For this review, take the finished solid that the model builds, in its own axes (mm). A direction names the side the tool comes from. Give positions to 0.01 mm unless a question says otherwise; leave off trailing zeros. Loops run counter-clockwise (first coordinate to the right, second up) from the corner with the lowest first, then second, coordinate; pieces in that order, holes last. Notation, with made-up numbers: (54.25, 20.25) -> (64.25, 20.25) arc R28 ccw to (64.25, 46.25) -> close; hole circle Ø8 at (43, 71.25). An arc over 180 degrees is marked (long way). One line per question, with ' | ' between items. Start each with the question number.
(1) Consider section D-D (z = 57). Write out the cut boundary in (x, y), and give its area (3 significant figures).
(2) Consider section B-B (x = -69). Write out the cut boundary in (y, z), and give its area (3 significant figures).
(3) Tool access review of faces 1 (the flat face through (-94.5, 38, 48)), 2 (the flat face through (-44, 30, 42)): name each direction out of +Z, -Z, +X, -X, +Y, -Y from which nothing blocks a thin tool from reaching the whole face with its end or side.
(4) Insertion check: P1, Ø12, axis at x = -35, y = 38.5, coming from the +Z side. The pin has a flat end and moves straight along its axis. Give the tip position at first contact, or say it passes through.
(5) Wall thickness on probe 1 along X at (y, z) = (80.5, 51.5); probe 2 along X at (y, z) = (29, 38); probe 3 along Y at (x, z) = (-86, 50.5): over which ranges is each line inside the solid? List them lowest first.
(6) Consider section C-C (y = 68). Write out the cut boundary in (x, z), and give its area (3 significant figures).
(7) Draft analysis for pull direction Y (two halves, no side actions). For faces 3 (the flat face through (0.5, 38, 48)), 4 (the flat face through (-93.5, 48, 51)), 5 (the flat face through (-48, -6, 48)), 6 (the flat face through (-48, 84, 48)), state which applies: +Y half, -Y half, draft (parallel to the pull), parting line (faces both ways), or undercut.
(8) Consider section A-A (z = 43.5). Write out the cut boundary in (x, y), and give its area (3 significant figures).
from build123d import *

# Parameters (mm, degrees)
SKETCH017_W    = 95
SKETCH017_H    = 90
PAD010_DEPTH   = 25
THICKNESS001_T = -1
SKETCH021_W    = 50
SKETCH021_H    = 70
PAD013_DEPTH   = 10


with BuildPart() as part:
    # Sketch017 → Pad010 (new body)
    with BuildSketch(Plane.XY):
        Rectangle(SKETCH017_W, SKETCH017_H)
    extrude(amount=PAD010_DEPTH)

    # Thickness001
    thickness001_openings = [part.faces().sort_by_distance(p)[0] for p in [
        (0, 0, 25),
    ]]
    offset(amount=THICKNESS001_T, openings=thickness001_openings)

    # Sketch021 (on DatumPlane) → Pad013 (join)
    with BuildSketch(Plane.XY.offset(1)):
        with Locations((-22, -9)):
            Rectangle(SKETCH021_W, SKETCH021_H)
    extrude(amount=PAD013_DEPTH)


with BuildPart() as part_1:
    # Body005 placement: moved
    add(part.part.moved(Location((-47, 39, 36))))


solid = part_1.part
A:
1) outline: (-94.5, -6) -> (0.5, -6) -> (0.5, 84) -> (-94.5, 84) -> close; hole (-93.5, -5) -> (-0.5, -5) -> (-0.5, 83) -> (-93.5, 83) -> close | area: 366 mm^2
2) outline: (-6, 36) -> (84, 36) -> (84, 61) -> (83, 61) -> (83, 37) -> (65, 37) -> (65, 47) -> (-5, 47) -> (-5, 61) -> (-6, 61) -> close | area: 838 mm^2
3) face 1: +Z, -Z, -X, +Y, -Y | face 2: +Z
4) P1: stops at z = 37
5) probe 1: x = -94.5 to -93.5, -0.5 to 0.5 | probe 2: x = -94.5 to -44, -0.5 to 0.5 | probe 3: y = -6 to -5, 83 to 84
6) outline: (-94.5, 36) -> (0.5, 36) -> (0.5, 61) -> (-0.5, 61) -> (-0.5, 37) -> (-93.5, 37) -> (-93.5, 61) -> (-94.5, 61) -> close | area: 143 mm^2
7) face 3: draft | face 4: undercut | face 5: -Y half | face 6: +Y half
8) outline: (-94.5, -6) -> (0.5, -6) -> (0.5, 84) -> (-94.5, 84) -> close; hole (-93.5, 65) -> (-44, 65) -> (-44, -5) -> (-0.5, -5) -> (-0.5, 83) -> (-93.5, 83) -> close | area: 3,830 mm^2
